For this review, take the finished solid that the model builds, in its own axes (mm). Face numbers are marked on the shaded views. A direction names the side the tool comes from. Give positions to 0.01 mm unless a question says otherwise; leave off trailing zeros. Write each loop counter-clockwise with the first axis right and the second up, starting at its lowest first coordinate (ties: lowest second). Pieces come first, ordered by that corner, then holes. Notation, with made-up numbers: M 37,-27 L 92,-27 A21 cw 92,-3 Z; hole C -2.75,9.5 d8. An arc over 180 degrees is marked long. One line per item, written item: value. Start each with the question number.
Item 1: Clearance check with flat-ended pins moving along their axes: pin 1 Ø9.5 at (x, z) = (-5, -14) entering from +Y; pin 2 Ø3 at (x, y) = (-10, 13) entering from -Z; pin 3 Ø9.5 at (x, y) = (-9, 17.5) entering from -Z. State where each tip first meets the part, or that it passes through.
Item 2: Consider section D-D, the plane x = -7. Write out the cut boundary in (y, z), and give its area (3 significant figures).
Item 3: Consider section A-A, the plane x = -10. Write out the cut boundary in (y, z).
Item 4: Consider section B-B, the plane y = 13. Write out the cut boundary in (x, z).
Item 5: To check wall thickness, follow probe 1 along X at (y, z) = (1.35, -13); probe 2 along Y at (x, z) = (-10, -1.7); probe 3 along Z at (x, y) = (-4.25, 7). State the ranges of each line that lie inside material, in increasing order.
Item 6: Consider section C-C, the plane z = -13. Write out the cut boundary in (x, y).
Item 7: Mouldability with a two-part tool opening along Y and no side actions: class the marked faces 3, 4 and 5 as released by +Y, released by -Y, zero draft, split by the parting line, or undercut.
Item 8: Tool access review of the marked faces 1 and 2: name each direction out of +Z, -Z, +X, -X, +Y, -Y from which nothing blocks a thin tool from reaching the whole face with its end or side.
```python
from build123d import *

# Parameters (mm, degrees)
BOSS_EXTRUDE1_DEPTH = 20
FILLET1_R           = 1
SKETCH3_R           = 2.5
CUT_EXTRUDE1_DEPTH  = 37.455452267
SKETCH4_R           = 2.5
CUT_EXTRUDE2_DEPTH  = 37.455452267


with BuildPart() as part:
    # Sketch2 → Boss-Extrude1 (new body)
    with BuildSketch(Plane(origin=(0, 0, 0), x_dir=(0, 0, -1), z_dir=(1, 0, 0))):
        with BuildLine():
            Line((1, 0), (23, 0))
            Line((23, 0), (23, 3))
            Line((23, 3), (4, 3))
            ThreePointArc((4, 3), (3.292893219, 3.292893219), (3, 4))
            Line((3, 4), (3, 23))
            Line((3, 23), (0, 23))
            Line((0, 23), (0, 1))
            ThreePointArc((0, 1), (0.292893219, 0.292893219), (1, 0))
        make_face()
    extrude(amount=-BOSS_EXTRUDE1_DEPTH)

    # Fillet1
    fillet1_edges = [part.edges().sort_by_distance(p)[0] for p in [
        (0, 1.5, -23),
        (-20, 23, -1.5),
        (-20, 1.5, -23),
        (0, 23, -1.5),
    ]]
    fillet(fillet1_edges, radius=FILLET1_R)

    # Sketch3 → Cut-Extrude1 (cut, through all)
    with BuildSketch(Plane(origin=(0, 0, -3), x_dir=(-1, 0, 0), z_dir=(0, 0, -1))):
        with Locations((10, 13)):
            Circle(SKETCH3_R)
    extrude(amount=-CUT_EXTRUDE1_DEPTH, mode=Mode.SUBTRACT)

    # Sketch4 → Cut-Extrude2 (cut, through all)
    with BuildSketch(Plane(origin=(0, 3, 0), x_dir=(1, 0, 0), z_dir=(0, 1, 0))):
        with Locations(Location((-10, 13, 0), (0, 0, 270))):
            Circle(SKETCH4_R)
    extrude(amount=-CUT_EXTRUDE2_DEPTH, mode=Mode.SUBTRACT)


solid = part.part
```
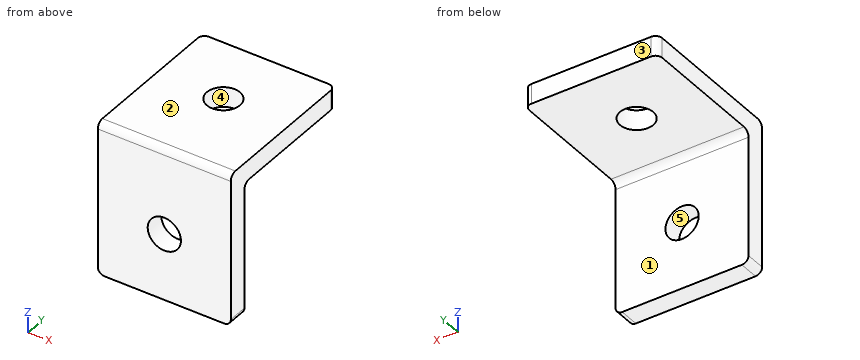
Model answer:
1. pin 1: stops at y = 3
1. pin 2: passes through
1. pin 3: stops at z = -3
2. outline: M 0,-23 L 3,-23 L 3,-4 A1 cw 4,-3 L 23,-3 L 23,0 L 1,0 A1 ccw 0,-1 Z
2. area: 129 mm2
3. outline: M 0,-23 L 3,-23 L 3,-15.5 L 0,-15.5 Z; M 0,-10.5 L 3,-10.5 L 3,-4 A1 cw 4,-3 L 10.5,-3 L 10.5,0 L 1,0 A1 ccw 0,-1 Z; M 15.5,-3 L 23,-3 L 23,0 L 15.5,0 Z
4. outline: M -20,-3 L -12.5,-3 L -12.5,0 L -20,0 Z; M -7.5,-3 L 0,-3 L 0,0 L -7.5,0 Z
5. probe 1: x = -20 to -12.5, -7.5 to 0
5. probe 2: y = 0 to 10.5, 15.5 to 23
5. probe 3: z = -3 to 0
6. outline: M -20,0 L -12.5,0 L -12.5,3 L -20,3 Z; M -7.5,0 L 0,0 L 0,3 L -7.5,3 Z
7. face 3: released by +Y
7. face 4: undercut
7. face 5: zero draft
8. face 1: -Z, +X, -X, +Y
8. face 2: +Z, +X, -X, +Y, -Y
